Drawing for the job (mm, zero at the part's lowest x, y, z). Give positions to 0.01 mm unless a question says otherwise; leave off trailing zeros. Loops run counter-clockwise (first coordinate to the right, second up) from the corner with the lowest first, then second, coordinate; pieces in that order, holes last. Notation, with made-up numbers: (42, -39) -> (82, -39) arc R36 ccw to (82, -5) -> close; hole circle Ø7 at (-22, -30.5). An arc over 180 degrees is marked (long way). Write item = value, one per line.
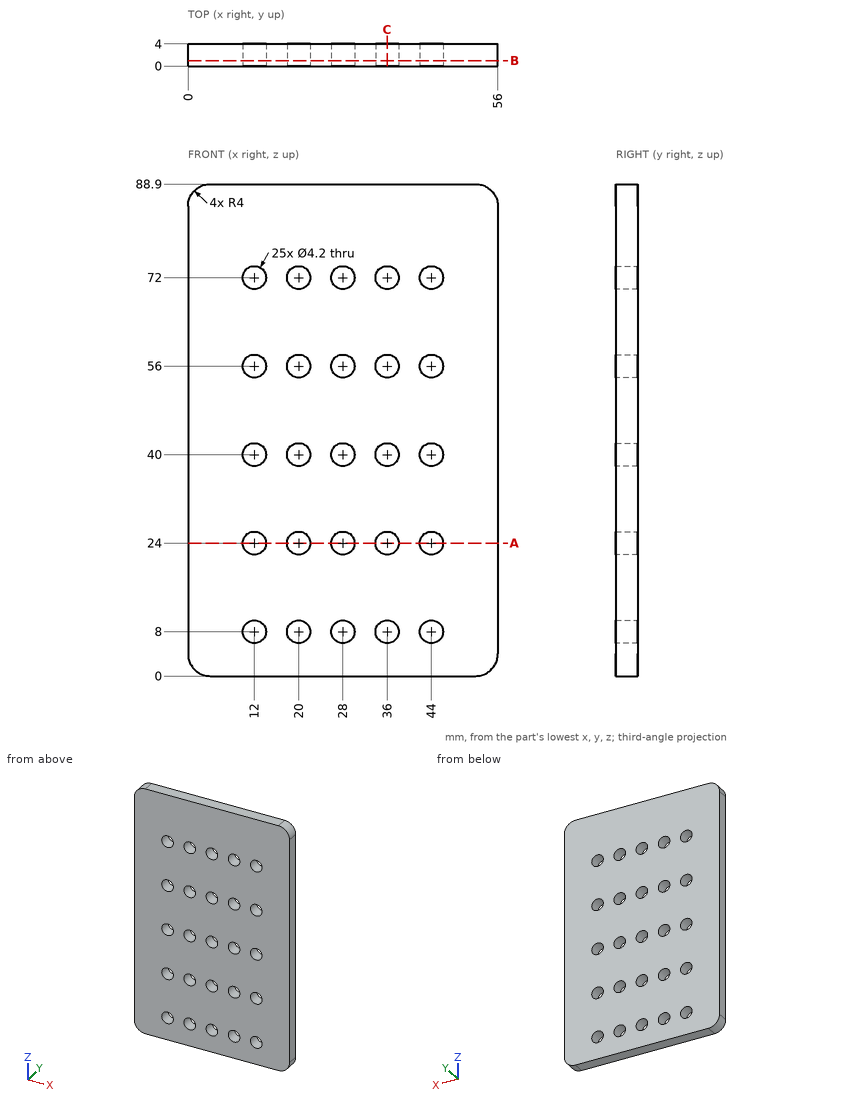
1) Slice it at B-B, the plane y = 1. Count the separate pieces of the cut face and the enclosed holes in it, and give its area (3 significant figures).
Resolved:
separate_pieces = 1
enclosed_holes = 25
area = 4,620 mm²
2) Slice it at C-C, the plane x = 36. List the corners of the cut face in (y, z).
Resolved:
outline = (0, 0) -> (4, 0) -> (4, 5.9) -> (0, 5.9) -> close; (0, 10.1) -> (4, 10.1) -> (4, 21.9) -> (0, 21.9) -> close; (0, 26.1) -> (4, 26.1) -> (4, 37.9) -> (0, 37.9) -> close; (0, 42.1) -> (4, 42.1) -> (4, 53.9) -> (0, 53.9) -> close; (0, 58.1) -> (4, 58.1) -> (4, 69.9) -> (0, 69.9) -> close; (0, 74.1) -> (4, 74.1) -> (4, 88.9) -> (0, 88.9) -> close
3) Slice it at A-A, the plane z = 24. List the corners of the cut face in (x, y).
Resolved:
outline = (0, 0) -> (9.9, 0) -> (9.9, 4) -> (0, 4) -> close; (14.1, 0) -> (17.9, 0) -> (17.9, 4) -> (14.1, 4) -> close; (22.1, 0) -> (25.9, 0) -> (25.9, 4) -> (22.1, 4) -> close; (30.1, 0) -> (33.9, 0) -> (33.9, 4) -> (30.1, 4) -> close; (38.1, 0) -> (41.9, 0) -> (41.9, 4) -> (38.1, 4) -> close; (46.1, 0) -> (56, 0) -> (56, 4) -> (46.1, 4) -> close
4) Drill centre line: line 1 along X through (y, z) = (3.05, 40). Where is it in solid material? Low to high. Write a range as [from, to].
Resolved:
line_1 = [0, 9.9], [14.1, 17.9], [22.1, 25.9], [30.1, 33.9], [38.1, 41.9], [46.1, 56]
